Autodesk Inventor part; units mm, degrees
ref_plane "YZ Plane" through (0, 0, 0) normal (1, 0, 0) x (0, 1, 0)
ref_plane "XZ Plane" through (0, 0, 0) normal (0, 1, 0) x (-1, 0, 0)
ref_plane "XY Plane" through (0, 0, 0) normal (0, 0, 1) x (1, 0, 0)
sketch "Sketch1" plane through (0, 0, 0) normal (0, 0, 1) x (1, 0, 0)
  line L0 (0, 0) -> (6, 0)
  line L1 (6, 0) -> (6, 71)
  line L2 (6, 71) -> (0, 71)
  line L3 (0, 71) -> (0, 0)
  line L4 (3, 0) -> (3, 3)
  circle A0 centre (3, 3) radius 1.425
  circle A1 centre (3, 3) radius 3
  line L5 (3, 71) -> (3, 68)
  circle A2 centre (3, 68) radius 1.425
  circle A3 centre (3, 68) radius 3
  point P0 (6, 3)
  point P1 (6, 68)
  point P2 (0, 68)
  point P3 (0, 3)
  dimension "d10" = 6
  dimension "d11" = 71
  dimension "d12" = 3
  dimension "d13" = 6
  dimension "d14" = 2.85
  dimension "d15" = 3
  dimension "d16" = 6
  dimension "d17" = 2.85
extrude "Extrusion1" add sketch "Sketch1" along normal blind 5 contours A1 | L3 A3 L1 A1 | A3
properties part number "Exoskeleton 1"
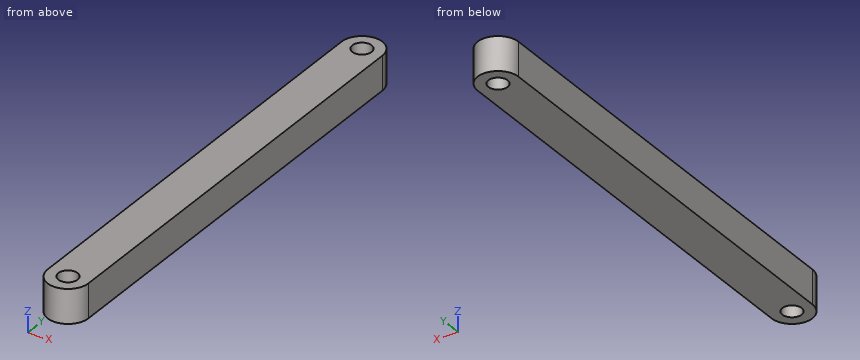
Source: CAD feature listing. Evaluate the final solid. Frame: model axes, mm. Give positions to 0.01 mm unless a question says otherwise; leave off trailing zeros. Order: outer loops, then holes, each group sorted by start corner. A loop starts at its lowest first (then second) coordinate and runs counter-clockwise, first axis right, second up. Notation, with made-up numbers: (66.25, -33.75) -> (121.25, -33.75) arc R27 ccw to (121.25, -17.75) -> close; hole circle Ø3 at (-5.5, 42.5). An arc over 180 degrees is marked (long way). Use a Markdown table: item, result.
Q1. Section A-A (x = 3). Return the cut outline in (y, z) (3 decimals), and give its area (4 significant figures).
A:
| item | result |
|---|---|
| outline | (0, 0) -> (1.575, 0) -> (1.575, 5) -> (0, 5) -> close; (4.425, 0) -> (66.575, 0) -> (66.575, 5) -> (4.425, 5) -> close; (69.425, 0) -> (71, 0) -> (71, 5) -> (69.425, 5) -> close |
| area | 326.5 mm^2 |
Q2. First-contact query: P1, Ø1.7, axis at x = 3, y = 68, coming from the -Z side; P2, Ø1, axis at x = 4, z = 0.5, coming from the -Y side. Flat tips, straight axial feed; report the tip coordinate or a pass-through.
A:
| item | result |
|---|---|
| P1 | through |
| P2 | y = 0.04 |
Q3. Material intervals for line 1 (Y direction, x = 3, z = 2.5) (3 decimals); line 2 (X direction, y = 68, z = 2.3) (3 decimals); line 3 (Y direction, x = 1.8, z = 2.55), sorted ascending. Write a range as [from, to].
A:
| item | result |
|---|---|
| line 1 | [0, 1.575], [4.425, 66.575], [69.425, 71] |
| line 2 | [0, 1.575], [4.425, 6] |
| line 3 | [0.25, 2.23], [3.77, 67.23], [68.77, 70.75] |
Q4. Section B-B (z = 4.1). Return the cut outline in (x, y) (3 decimals), and give its area (3 significant figures).
A:
| item | result |
|---|---|
| outline | (0, 3) arc R3 ccw to (6, 3) -> (6, 68) arc R3 ccw to (0, 68) -> close; hole circle Ø2.85 at (3, 3); hole circle Ø2.85 at (3, 68) |
| area | 406 mm^2 |
